Here's how the part is built. I have some questions about the finished solid (model axes, mm). Face numbers are marked on the shaded views. A direction names the side the tool comes from. Round coordinates to 2 decimals unless told otherwise and drop trailing zeros. Loops run counter-clockwise (first coordinate to the right, second up) from the corner with the lowest first, then second, coordinate; pieces in that order, holes last. Notation, with made-up numbers: (9.5, 72) -> (47.5, 72) arc R19 cw to (47.5, 102) -> close; hole circle Ø1 at (37, 33). An arc over 180 degrees is marked (long way). One line per item, written item: value. Start each with the question number.
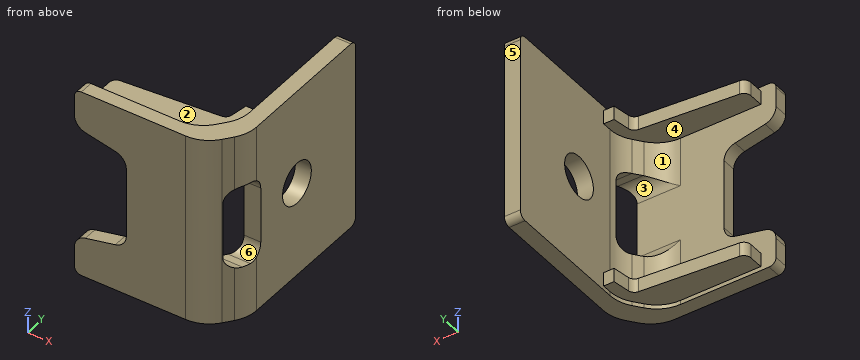
```python
from build123d import *

# Parameters (mm, degrees)
F1_DEPTH  = 27.5
F2_W      = 5.1
F2_H      = 12.1
F2_R      = 3
F3_DEPTH  = 12.5
F4_W      = 7.5
F4_H      = 2
F5_DEPTH  = 17.5
F7_DEPTH  = 26.901
F8_R      = 1
F9_R      = 2
F11_DEPTH = 26.901
F12_R     = 2


with BuildPart() as f1:
    # F0 (on Top) → F1 (new body)
    with BuildSketch(Plane.XY):
        with BuildLine():
            Line((0, 2), (0, 0))
            Line((0, 0), (16.0545809717, 0))
            ThreePointArc((16.0545809717, 0), (18.2513382025, 0.5084236989), (20.0013420586, 1.9302969324))
            Line((20.0013420586, 1.9302969324), (20.9467610869, 3.1458356831))
            ThreePointArc((20.9467610869, 3.1458356831), (21.7293659953, 4.5928566245), (22, 6.2155387507))
            Line((22, 6.2155387507), (22, 26.9))
            Line((22, 26.9), (19.7, 26.9))
            Line((19.7, 26.9), (19.7, 8.1448620011))
            ThreePointArc((19.7, 8.1448620011), (19.4293659953, 6.5221798749), (18.6467610869, 5.0751589336))
            Line((18.6467610869, 5.0751589336), (17.7563128638, 3.9302969324))
            ThreePointArc((17.7563128638, 3.9302969324), (16.0063090077, 2.5084236989), (13.8095517769, 2))
            Line((13.8095517769, 2), (0, 2))
        make_face()
    extrude(amount=F1_DEPTH)

    # F2 (on face) → F3 (cut, symmetric)
    with BuildSketch(Plane(origin=(19.7, 0, 0), x_dir=(0, -1, 0), z_dir=(-1, 0, 0))):
        with Locations((-4.55, 13.75)):
            Rectangle(F2_W, F2_H)
        with Locations((-14.65, 13.75)):
            Circle(F2_R)
    extrude(amount=F3_DEPTH, both=True, mode=Mode.SUBTRACT)

    # F4 (on face) → F5 (join)
    with BuildSketch(Plane(origin=(19.7, 0, 0), x_dir=(0, -1, 0), z_dir=(-1, 0, 0))):
        with Locations((-5.75, 25.9)):
            Rectangle(F4_W, F4_H)
        with Locations((-5.75, 1.6)):
            Rectangle(F4_W, F4_H)
    extrude(amount=F5_DEPTH)

    # F6 (on face) → F7 (cut, through all)
    with BuildSketch(Plane(origin=(0, 0, 0.6), x_dir=(1, 0, 0), z_dir=(0, 0, -1))):
        Polygon((17.7, -6.3), (2.2, -5), (2.2, -9.5), (18.2, -9.5), align=None)
    extrude(amount=-F7_DEPTH, mode=Mode.SUBTRACT)

    # F8
    f8_edges = [f1.edges().sort_by_distance(p)[0] for p in [
        (2.2, 5, 1.6),
        (2.2, 5, 25.9),
        (0, 1, 0),
        (0, 1, 27.5),
        (20.85, 26.9, 0),
        (20.85, 26.9, 27.5),
        (17.7, 6.3, 1.6),
        (17.7, 6.3, 25.9),
    ]]
    fillet(f8_edges, radius=F8_R)

    # F9
    f9_edges = [f1.edges().sort_by_distance(p)[0] for p in [
        (16.932554, 2, 19.8),
        (20.794804, 7.1, 19.8),
        (16.932554, 2, 7.7),
        (20.794804, 7.1, 7.7),
    ]]
    fillet(f9_edges, radius=F9_R)

    # F10 (on face) → F11 (cut, through all)
    with BuildSketch(Plane.XZ):
        Polygon((0, 22), (0, 5.5), (7.5, 7.1), (7.5, 20.4), align=None)
    extrude(amount=-F11_DEPTH, mode=Mode.SUBTRACT)

    # F12
    f12_edges = [f1.edges().sort_by_distance(p)[0] for p in [
        (0, 1, 5.5),
        (0, 1, 22),
        (7.5, 1, 20.4),
        (7.5, 1, 7.1),
    ]]
    fillet(f12_edges, radius=F12_R)


solid = f1.part
```
Q1. Which directions (+Z, -Z, +X, -X, +Y, -Y) give clear straight access to the entire face, cutting with the end or side of a thin tool? Please do the marked faces 1, 2 and 3.
Q2. I want a section at C-C on x = 3.5. Please give me the cut outline in (y, z), plus the area to 3 significant figures.
Q3. Will these pins go through, and if not, where does the flat tip stop? P1, Ø10, axis at x = 5, y = 3, coming from the +Z side; P2, Ø0.6, axis at y = 3, z = 2, coming from the -X side; P3, Ø15, axis at y = 19.5, z = 17, coming from the -X side; P4, Ø1.5, axis at x = 18, z = 11.5, coming from the -Y side (3 decimals).
Q4. I want a section at B-B on z = 13.75. Please give me the cut outline in (x, y), plus the area to 3 significant figures.
Q5. If I drill on line 1 along Z through (x, y) = (20.4, 14.65); line 2 along Z through (x, y) = (6.5, 2.75); line 3 along Y through (x, z) = (2.25, 3), over which ranges is the centre line in solid material (lowest first)?
Q6. I want a section at D-D on x = 11.5. Please give me the cut outline in (y, z), plus the area to 3 significant figures.
Q7. I want a section at A-A on y = 14.65. Please give me the cut outline in (x, z), plus the area to 4 significant figures.
Q8. If we mould it in two halves opening along Y, with no side actions, what happens to the marked faces 4, 5 and 6? For each: released by +Y, released by -Y, zero draft, split by the parting line, or undercut.
Answers below:
1. face 1: -X, +Y
1. face 2: +Z, -X, +Y
1. face 3: +X, -X
2. outline: (0, 0) -> (2, 0) -> (2, 0.6) -> (5.11, 0.6) -> (5.11, 2.6) -> (2, 2.6) -> (2, 6.25) -> (0, 6.25) -> close; (0, 21.25) -> (2, 21.25) -> (2, 24.9) -> (5.11, 24.9) -> (5.11, 26.9) -> (2, 26.9) -> (2, 27.5) -> (0, 27.5) -> close
2. area: 37.4 mm^2
3. P1: stops at z = 27.5
3. P2: stops at x = 2.2
3. P3: stops at x = 19.7
3. P4: stops at y = 0.145
4. outline: (7.5, 0) -> (16.05, 0) arc R5 ccw to (20, 1.93) -> (20.06, 2) -> (7.5, 2) -> close; (19.59, 7.1) -> (22, 7.1) -> (22, 11.65) -> (19.7, 11.65) -> (19.7, 8.14) arc R5 cw to start; (19.7, 17.65) -> (22, 17.65) -> (22, 26.9) -> (19.7, 26.9) -> close
4. area: 54.5 mm^2
5. line 1: z = 0 to 10.75, 16.75 to 27.5
5. line 2: z = 0.6 to 2.6, 24.9 to 26.9
5. line 3: y = 0 to 2
6. outline: (0, 0) -> (2, 0) -> (2, 0.6) -> (5.78, 0.6) -> (5.78, 2.6) -> (2, 2.6) -> (2, 24.9) -> (5.78, 24.9) -> (5.78, 26.9) -> (2, 26.9) -> (2, 27.5) -> (0, 27.5) -> close
6. area: 70.1 mm^2
7. outline: (19.7, 0) -> (22, 0) -> (22, 10.75) -> (19.7, 10.75) -> close; (19.7, 16.75) -> (22, 16.75) -> (22, 27.5) -> (19.7, 27.5) -> close
7. area: 49.45 mm^2
8. face 4: zero draft
8. face 5: released by +Y
8. face 6: undercut
